Here's how the part is built. I have some questions about the finished solid (model axes, mm). A direction names the side the tool comes from. Round coordinates to 2 decimals unless told otherwise and drop trailing zeros. Order: outer loops, then holes, each group sorted by start corner. A loop starts at its lowest first (then second) coordinate and runs counter-clockwise, first axis right, second up. Notation, with made-up numbers: (22.25, -35) -> (77.25, -35) arc R26 cw to (77.25, -21) -> close; hole circle Ø3 at (-37.75, 86). An arc over 180 degrees is marked (long way). Use a Markdown table: item, result. Add a question column.
Autodesk Inventor part; units mm, degrees
ref_plane "YZ Plane" through (0, 0, 0) normal (1, 0, 0) x (0, 1, 0)
ref_plane "XZ Plane" through (0, 0, 0) normal (0, 1, 0) x (-1, 0, 0)
ref_plane "XY Plane" through (0, 0, 0) normal (0, 0, 1) x (1, 0, 0)
sketch "Náčrt1" plane through (0, 0, 0) normal (0, 0, 1) x (1, 0, 0)
  line L0 (0, 35) -> (0, -35)
  line L1 (-59.5, 0) -> (59.5, 0)
  line L2 (42.5, -25) -> (-42.5, -25)
  line L3 (-42.5, -25) -> (-42.5, 25)
  line L4 (-42.5, 25) -> (42.5, 25)
  line L5 (42.5, 25) -> (42.5, -25)
  point P0 (0, 0)
  dimension "d1" = 85
  dimension "d2" = 50
extrude "Vysunutí1" add sketch "Náčrt1" along normal blind 3
sketch "Náčrt2" plane through (0, 0, 0) normal (0, 0, -1) x (-1, 0, 0)
  line L0 (-42.5, 25) -> (42.5, 25)
  line L1 (-42.5, -25) -> (-42.5, 25)
  line L2 (42.5, -25) -> (-42.5, -25)
  line L3 (42.5, 25) -> (42.5, -25)
  line L4 (45, 27.5) -> (-45, 27.5)
  line L5 (-45, 27.5) -> (-45, -27.5)
  line L6 (-45, -27.5) -> (45, -27.5)
  line L7 (45, -27.5) -> (45, 27.5)
  line L8 (-42.5, 25) -> (42.5, 25)
  line L9 (42.5, 25) -> (42.5, -25)
  line L10 (42.5, -25) -> (-42.5, -25)
  line L11 (-42.5, -25) -> (-42.5, 25)
  point P0 (0, 0)
  dimension "d5" = 2.5
extrude "Vysunutí2" add sketch "Náčrt2" against normal blind 30
sketch "Náčrt3" plane through (0, 0, 3) normal (0, 0, 1) x (1, 0, 0)
  line L0 (42.5, 25) -> (-42.5, 25)
  line L1 (-42.5, 25) -> (-42.5, -25)
  line L2 (-42.5, -25) -> (42.5, -25)
  line L3 (42.5, -25) -> (42.5, 25)
  line L4 (0, 35) -> (0, -35)
  line L5 (-63, 0) -> (63, 0)
  line L6 (2.5, 21.5) -> (37.5, 21.5) construction
  line L7 (37.5, 21.5) -> (37.5, -21.5) construction
  line L8 (37.5, -21.5) -> (2.5, -21.5) construction
  line L9 (2.5, -21.5) -> (2.5, 21.5) construction
  line L10 (-2.5, 21.5) -> (-37.5, 21.5) construction
  line L11 (-37.5, 21.5) -> (-37.5, -21.5) construction
  line L12 (-37.5, -21.5) -> (-2.5, -21.5) construction
  line L13 (-2.5, -21.5) -> (-2.5, 21.5) construction
  circle A0 centre (6.5, 16) radius 1
  circle A1 centre (6.5, -16) radius 1
  circle A2 centre (-6.5, 16) radius 1
  circle A3 centre (-6.5, -16) radius 1
  point P0 (0, 0)
  point P1 (9, -16)
  dimension "d8" = 35
  dimension "d9" = 43
  dimension "d10" = 3.5
  dimension "d11" = 5
  dimension "d15" = 2
  dimension "d16" = 36
  dimension "d17" = 16
extrude "Vysunutí3" add sketch "Náčrt3" along normal blind 5 contours A0 | A1 | A2 | A3
sketch "Náčrt4" plane through (45, -27.5, 0) normal (1, 0, 0) x (0, 0, -1)
  line L0 (-3, 2.5) -> (-3, 52.5)
  line L1 (0, 55) -> (0, 0)
  line L2 (0, 55) -> (-30, 55)
  line L3 (-30, 0) -> (-30, 55)
  line L4 (0, 0) -> (-30, 0)
  line L5 (-36, 27.5) -> (6, 27.5)
  line L6 (0, -11) -> (0, 66)
  line L7 (-7, 34) -> (-15, 34)
  line L8 (-15, 34) -> (-15, 49)
  line L9 (-15, 49) -> (-7, 49)
  line L10 (-7, 49) -> (-7, 34)
  point P0 (0, 27.5)
  point P1 (-3, 34)
  point P2 (-3, 49)
  dimension "d20" = 8
  dimension "d21" = 15
  dimension "d22" = 6
  dimension "d24" = 7
extrude "Vysunutí4" cut sketch "Náčrt4" against normal up to surface (2.5 mm away) contours L7 L8 L9 L10
pattern_circular "Kruhové pole1" count 2 over 360 about axis through (0, 0, -10) along (0, 0, 1) of "Vysunutí4"
sketch "Náčrt5" plane through (-45, 27.5, 0) normal (0, 1, 0) x (1, 0, 0)
  line L0 (0, 0) -> (90, 0)
  line L1 (0, 0) -> (0, -30)
  line L2 (90, -30) -> (0, -30)
  line L3 (90, 0) -> (90, -30)
  line L4 (-18, 0) -> (108, 0)
  line L5 (45, 6) -> (45, -36)
  line L6 (37.5, -30) -> (52.5, -30)
  line L7 (52.5, -30) -> (52.5, -107)
  line L8 (52.5, -107) -> (37.5, -107)
  line L9 (37.5, -107) -> (37.5, -30)
  line L10 (0, 0) -> (90, 0)
  line L11 (52.5, -30) -> (37.5, -30)
  line L12 (37.5, -30) -> (37.5, 0)
  line L13 (37.5, 0) -> (52.5, 0)
  line L14 (52.5, 0) -> (52.5, -30)
  point P0 (45, 0)
  dimension "d31" = 77
  dimension "d32" = 15
  dimension "d33" = 15
extrude "Vysunutí5" add sketch "Náčrt5" along normal mid plane 5 contours L0 L5 L2 L12 | L0 L14 L2 L5 | L2 L7 L8 L9
fillet "Zaoblení1" radius 2 4 edges at (-45, 27.5, 15) (-45, -27.5, 15) (45, -27.5, 15) (45, 27.5, 15)
sketch "Náčrt6" plane through (-45, 30, 0) normal (0, 1, 0) x (1, 0, 0)
  line L0 (37.5, -107) -> (52.5, -107)
  line L1 (52.5, -107) -> (52.5, 0)
  line L2 (52.5, 0) -> (37.5, 0)
  line L3 (37.5, 0) -> (37.5, -107)
  point P0 (45, 0)
  point P1 (45, -92)
  point P2 (45, -107)
  dimension "d37" = 7.5
  dimension "d38" = 15
hole "Díra1" at (0, 30, 92) direction (0, -1, 0) diameter 6.6 end through all
chamfer "Zkosení1" distance 2 angle 45 3 edges at (7.5, 30, 53.5) (-7.5, 30, 53.5) (0, 30, 107)
properties part number "adapter_box_3D tisk"
(1) I'm going to push flat-ended pins straight in: P1, Ø1.2, axis at x = -44.5, z = 11.5, coming from the -Y side; P2, Ø1.5, axis at x = -6.5, z = 62, coming from the +Y side; P3, Ø1.2, axis at x = 44, y = 14.5, coming from the -Z side; P4, Ø2, axis at x = -43.5, z = 12.5, coming from the +Y side. Where does each tip first touch, or does it pass through?
(2) I want a section at B-B on y = 13.5. List the corners of the cut face in (x, z) for me.
(3) On a 3-axis mill with a long thin cutter (end or side, diameter ignored), from which of +Z, -Z, +X, -X, +Y, -Y can I reach the whole of each face in a straight line? I mean faces 5 (the flat face through (0, 25, 35)), 6 (the flat face through (44, 21.5, 11)), 7 (the flat face through (-44, -14, 15)), 8 (the flat face through (1, -27.5, 15)), 9 (the flat face through (-25, 27.5, 15)). Say none if no direction works.
(4) I want a section at A-A on x = 0. List the corners of the cut face in (y, z) for me, and give its area (3 significant figures).
(5) Please list where these lines run through material, in increasing order: probe 1 along Z at (x, y) = (0, 27.3); probe 2 along X at (y, z) = (28, 92); probe 3 along X at (y, z) = (15, 23.5). Write a range as from..to.
(6) I want a section at C-C on z = 92. List the corners of the cut face in (x, y) for me, and give its area (3 significant figures).
(7) I want a section at D-D on z = 27. List the corners of the cut face in (x, y) for me.
(8) If we mould it in two halves opening along X, with no side actions, what happens to faces 1 (the flat face through (-44, -6.5, 11)), 2 (the flat face through (-1, -25, 16)), 3 (the cylindrical face through (-0.1, 27.5, 88.7)), 4 (the flat face through (45, 0, 15))? For each: pulls with the +X half, pulls with the -X half, needs draft (parallel to the pull), parting line crosses it, or undercut.
Output:
| question | item | result |
|---|---|---|
| 1 | P1 | y = -27.29 |
| 1 | P2 | y = 29.75 |
| 1 | P3 | z = 0 |
| 1 | P4 | y = 27.5 |
| 2 | outline | (-45, 0) -> (45, 0) -> (45, 7) -> (42.5, 7) -> (42.5, 3) -> (-42.5, 3) -> (-42.5, 30) -> (-45, 30) -> close; (42.5, 15) -> (45, 15) -> (45, 30) -> (42.5, 30) -> close |
| 3 | face 5 | +Z |
| 3 | face 6 | +X |
| 3 | face 7 | -X |
| 3 | face 8 | +Z, -Z, +X, -X, -Y |
| 3 | face 9 | +Z, -Z, -X, +Y |
| 4 | outline | (-27.5, 0) -> (30, 0) -> (30, 88.7) -> (25, 88.7) -> (25, 3) -> (-25, 3) -> (-25, 30) -> (-27.5, 30) -> close; (25, 95.3) -> (30, 95.3) -> (30, 105) -> (28, 107) -> (25, 107) -> close |
| 4 | area | 725 mm² |
| 5 | probe 1 | 0..88.7, 95.3..107 |
| 5 | probe 2 | -7.5..-3.3, 3.3..7.5 |
| 5 | probe 3 | -45..-42.5, 42.5..45 |
| 6 | outline | (-7.5, 25) -> (-3.3, 25) -> (-3.3, 30) -> (-5.5, 30) -> (-7.5, 28) -> close; (3.3, 25) -> (7.5, 25) -> (7.5, 28) -> (5.5, 30) -> (3.3, 30) -> close |
| 6 | area | 38.0 mm² |
| 7 | outline | (-45, -25.5) arc R2 ccw to (-43, -27.5) -> (43, -27.5) arc R2 ccw to (45, -25.5) -> (45, 25.5) arc R2 ccw to (43, 27.5) -> (7.5, 27.5) -> (7.5, 28) -> (5.5, 30) -> (-5.5, 30) -> (-7.5, 28) -> (-7.5, 27.5) -> (-43, 27.5) arc R2 ccw to (-45, 25.5) -> close; hole (-42.5, -25) -> (42.5, -25) -> (42.5, 25) -> (-42.5, 25) -> close |
| 8 | face 1 | needs draft |
| 8 | face 2 | undercut |
| 8 | face 3 | undercut |
| 8 | face 4 | pulls with the +X half |
